from build123d import *

# Parameters (mm, degrees)
SKETCH1_W           = 11.5
SKETCH1_H           = 7
BOSS_EXTRUDE1_DEPTH = 100
M5_TAPPED_HOLE1_D   = 4.2


with BuildPart() as part:
    # Sketch1 → Boss-Extrude1 (new, symmetric)
    with BuildSketch(Plane.XY):
        Rectangle(SKETCH1_W, SKETCH1_H)
    extrude(amount=BOSS_EXTRUDE1_DEPTH, both=True)

    # M5 Tapped Hole1 (through all)
    with Locations(Plane(origin=(0, 3.5, 0), x_dir=(1, 0, 0), z_dir=(0, 1, 0))):
        with Locations((0, 90), (0, 30), (0, -30), (0, -90)):
            Hole(M5_TAPPED_HOLE1_D / 2)


solid = part.part
Can you work these out from the model? Positions are in its coordinate system, mm. Give positions to 0.01 mm unless a question says otherwise; leave off trailing zeros. Loops run counter-clockwise (first coordinate to the right, second up) from the corner with the lowest first, then second, coordinate; pieces in that order, holes last. Notation, with made-up numbers: (64, 82) - (102, 82) arc R24 ccw to (102, 93) - close; hole circle Ø8 at (-27.75, -6.75). An arc over 180 degrees is marked (long way). Return JSON: item names as keys, results as strings.
1. I want a section at C-C on y = 0. Please give me the cut outline in (x, z).
Output values:
{"outline": "(-5.75, -100) - (5.75, -100) - (5.75, 100) - (-5.75, 100) - close; hole circle Ø4.2 at (0, -90); hole circle Ø4.2 at (0, -30); hole circle Ø4.2 at (0, 30); hole circle Ø4.2 at (0, 90)"}
2. We'd pull the mould along Z, two halves only. Please class faces 1 (the face through (-0.969, -0.049, 31.863)), 2 (the face through (0, -3.5, 1)), 3 (the face through (0, 0, 100)), 4 (the face through (0, 0, -100)): +Z half, -Z half, draft (parallel to the pull), parting line (faces both ways), or undercut.
Output values:
{"face 1": "undercut", "face 2": "draft", "face 3": "+Z half", "face 4": "-Z half"}
3. I'm going to push a flat-ended pin straight in: pin 1 Ø3.5 at (x, z) = (0, 90) entering from -Y. Where does the tip first touch, or does it pass through?
Output values:
{"pin 1": "passes through"}
4. I want a section at B-B on x = 0. Please give me the cut outline in (y, z), and give its area (3 significant figures).
Output values:
{"outline": "(-3.5, -100) - (3.5, -100) - (3.5, -92.1) - (-3.5, -92.1) - close; (-3.5, -87.9) - (3.5, -87.9) - (3.5, -32.1) - (-3.5, -32.1) - close; (-3.5, -27.9) - (3.5, -27.9) - (3.5, 27.9) - (-3.5, 27.9) - close; (-3.5, 32.1) - (3.5, 32.1) - (3.5, 87.9) - (-3.5, 87.9) - close; (-3.5, 92.1) - (3.5, 92.1) - (3.5, 100) - (-3.5, 100) - close", "area": "1,280 mm²"}
5. If I drill on line 1 (Z direction, x = 0, y = -0.25); line 2 (X direction, y = -1, z = -30); line 3 (Z direction, x = 1.5, y = -2), over which ranges is the centre line in solid material (lowest first)?
Output values:
{"line 1": "z = -100 to -92.1, -87.9 to -32.1, -27.9 to 27.9, 32.1 to 87.9, 92.1 to 100", "line 2": "x = -5.75 to -2.1, 2.1 to 5.75", "line 3": "z = -100 to -91.47, -88.53 to -31.47, -28.53 to 28.53, 31.47 to 88.53, 91.47 to 100"}
6. I want a section at A-A on z = -30. Please give me the cut outline in (x, y).
Output values:
{"outline": "(-5.75, -3.5) - (-2.1, -3.5) - (-2.1, 3.5) - (-5.75, 3.5) - close; (2.1, -3.5) - (5.75, -3.5) - (5.75, 3.5) - (2.1, 3.5) - close"}
